Model file for the job. Use its own axes, mm. A direction names the side the tool comes from. Round coordinates to 2 decimals unless told otherwise and drop trailing zeros. Loops run counter-clockwise (first coordinate to the right, second up) from the corner with the lowest first, then second, coordinate; pieces in that order, holes last. Notation, with made-up numbers: M -25,69.25 L 32,69.25 A11 ccw 32,83.25 Z; hole C 28.25,-15.5 d3. An arc over 180 degrees is marked long. Use a Markdown table: item, result. Add a question column.
Item 1: Pin check, flat tip, straight feed: P1, Ø5.5, axis at x = -23.5, z = -11.5, coming from the +Y side. Stop position of the tip, or through.
Item 2: Saw through at A-A on x = 0. Write the cut outline in (y, z).
Item 3: Wall check: L1, parallel to X at y = 0.5, z = -11.5; L2, parallel to Y at x = 7, z = -23; L3, parallel to Y at x = 4.5, z = -19.5. Give the ranges that are in metal, low to high. Write a range as from..to.
Item 4: Tool access for faces 1 (the flat face through (0, -29, 0)), 2 (the flat face through (5.27, 4, -14.79)): list every direction of +Z, -Z, +X, -X, +Y, -Y with a clear straight run to the whole face (end or side of a thin tool).
Item 5: Two-plate mould, pull along Z, no slides. Class faces 3 (the cylindrical face through (28, -29.37, -1.43)), 4 (the cylindrical face through (28.07, -30.63, -28.5)), 5 (the flat face through (0, -15, -10)), 6 (the cylindrical face through (26.47, 0.21, -11.96)): +Z half, -Z half, draft (parallel to the pull), parting line (faces both ways), or undercut.
Item 6: Saw through at B-B on x = -23. Write the cut outline in (y, z), then the cut area to 3 significant figures.
```python
from build123d import *

# Parameters (mm, degrees)
SKETCH1_W           = 59
SKETCH1_H           = 30
BOSS_EXTRUDE1_DEPTH = 30
SKETCH2_R           = 2.5
SKETCH2_R_2         = 3.5
CUT_EXTRUDE1_DEPTH  = 52.674461778
SKETCH3_W           = 59
SKETCH3_H           = 60
BOSS_EXTRUDE2_DEPTH = 30
FILLET1_R           = 5
FILLET2_R           = 5
FILLET3_R           = 5
FILLET4_R           = 5


with BuildPart() as part:
    # Sketch1 → Boss-Extrude1 (new body)
    with BuildSketch(Plane.XY):
        Rectangle(SKETCH1_W, SKETCH1_H)
        Polygon((4, 2.727207794), (6.572792206, 5.3), (8, 5.3), (8, 3.1), (10, 5.1), (10, 10), (5.1, 10), (3.1, 8), (5.3, 8), (5.3, 6.572792206), (2.727207794, 4), (-2.727207794, 4), (-5.3, 6.572792206), (-5.3, 8), (-3.1, 8), (-5.1, 10), (-10, 10), (-10, 5.1), (-8, 3.1), (-8, 5.3), (-6.572792206, 5.3), (-4, 2.727207794), (-4, -2.727207794), (-6.572792206, -5.3), (-8, -5.3), (-8, -3.1), (-10, -5.1), (-10, -10), (-5.1, -10), (-3.1, -8), (-5.3, -8), (-5.3, -6.572792206), (-2.727207794, -4), (2.727207794, -4), (5.3, -6.572792206), (5.3, -8), (3.1, -8), (5.1, -10), (10, -10), (10, -5.1), (8, -3.1), (8, -5.3), (6.572792206, -5.3), (4, -2.727207794), align=None, mode=Mode.SUBTRACT)
    extrude(amount=-BOSS_EXTRUDE1_DEPTH)

    # Sketch2 → Cut-Extrude1 (cut, through all)
    with BuildSketch(Plane(origin=(0, 15, 0), x_dir=(1, 0, 0), z_dir=(0, 1, 0))):
        with Locations(Location((0, 10, 0), (0, 0, 270))):
            Circle(SKETCH2_R)
        with Locations(Location((0, 20, 0), (0, 0, 270))):
            Circle(SKETCH2_R)
        with Locations(Location((23, 11.5, 0), (0, 0, 270))):
            Circle(SKETCH2_R_2)
        with Locations(Location((-23, 11.5, 0), (0, 0, 270))):
            Circle(SKETCH2_R_2)
    extrude(amount=-CUT_EXTRUDE1_DEPTH, mode=Mode.SUBTRACT)

    # Sketch3 → Boss-Extrude2 (add)
    with BuildSketch(Plane.XY):
        with Locations((0, -45)):
            Rectangle(SKETCH3_W, SKETCH3_H)
    extrude(amount=-BOSS_EXTRUDE2_DEPTH)

    # Fillet1
    fillet1_edges = [part.edges().sort_by_distance(p)[0] for p in [
        (29.5, -30, 0),
    ]]
    fillet(fillet1_edges, radius=FILLET1_R)

    # Fillet2
    fillet2_edges = [part.edges().sort_by_distance(p)[0] for p in [
        (29.5, -30, -30),
    ]]
    fillet(fillet2_edges, radius=FILLET2_R)

    # Fillet3
    fillet3_edges = [part.edges().sort_by_distance(p)[0] for p in [
        (-29.5, -30, -30),
    ]]
    fillet(fillet3_edges, radius=FILLET3_R)

    # Fillet4
    fillet4_edges = [part.edges().sort_by_distance(p)[0] for p in [
        (-29.5, -30, 0),
    ]]
    fillet(fillet4_edges, radius=FILLET4_R)


solid = part.part
```
Entries:
| question | item | result |
|---|---|---|
| 1 | P1 | y = -15 |
| 2 | outline | M -75,-30 L -4,-30 L -4,-22.5 L -15,-22.5 L -15,-17.5 L -4,-17.5 L -4,-12.5 L -15,-12.5 L -15,-7.5 L -4,-7.5 L -4,0 L -75,0 Z; M 4,-30 L 15,-30 L 15,-22.5 L 4,-22.5 Z; M 4,-17.5 L 15,-17.5 L 15,-12.5 L 4,-12.5 Z; M 4,-7.5 L 15,-7.5 L 15,0 L 4,0 Z |
| 3 | L1 | -29.5..-26.5, -19.5..-4, 4..19.5, 26.5..29.5 |
| 3 | L2 | -75..-10, -5.3..5.3, 10..15 |
| 3 | L3 | -75..-9.4, -8..-5.77, -3.23..3.23, 5.77..8, 9.4..15 |
| 4 | face 1 | +Z, +X, -X, +Y, -Y |
| 4 | face 2 | +Z, -Z |
| 5 | face 3 | +Z half |
| 5 | face 4 | -Z half |
| 5 | face 5 | undercut |
| 5 | face 6 | undercut |
| 6 | outline | M -75,-30 L 15,-30 L 15,-15 L -15,-15 L -15,-8 L 15,-8 L 15,0 L -75,0 Z |
| 6 | area | 2,490 mm2 |
